Input: part model. Units: mm. Frame: model coordinates. A direction names the side the tool comes from. Coordinates: 2 decimals unless noted, no trailing zeros. Loops run counter-clockwise (first coordinate to the right, second up) from the corner with the lowest first, then second, coordinate; pieces in that order, holes last.
(1) Section B-B, the plane z = 5. Return loops of the section in (x, y), then the cut area to 3 significant figures.
(2) Section C-C, the plane y = -16. Return loops of the section in (x, z), then the cut area to 3 significant figures.
(3) Set-up query: faces 4 (the face through (-31, -13, -23.456)), 5 (the face through (0, -32, 65.444)), 6 (the face through (0, 0.98, 91)). Return all of +Z, -Z, +X, -X, +Y, -Y with unobstructed straight access to the full face (end or side cutting, diameter ignored); none if empty.
(4) Mould query, pull axis Y, two halves, no side actions, for faces 1 (the face through (0, 0, 9)), 2 (the face through (0, -13, -48.856)), 3 (the face through (-13.68, -13, 91)). Classes: released by +Y, released by -Y, zero draft, split by the parting line, or undercut.
(5) Section A-A, the plane x = -2.5. Return loops of the section in (y, z), then the cut area to 3 significant figures.
(6) Line query: L1, parallel to Z at x = 35, y = -22; L2, parallel to Z at x = 25, y = -25; L3, parallel to X at y = -10.5, z = 87.5. Output: solid intervals per line, ascending.
(7) Contact query for flat-ended pins moving along their axis: P1, Ø12, axis at y = -25, z = 89, coming from the -X side; P2, Ø12, axis at x = -7, z = -17, coming from the -Y side; P3, Ø1, axis at y = 8.5, z = 68.5, coming from the +X side. Output: stop coordinate, or through.
```python
from build123d import *

# Parameters (mm, degrees)
F1_DEPTH = 25.4
F2_R     = 7.890546565
F3_DEPTH = 63.501
F5_DEPTH = 50.8
F7_DEPTH = 50.8


with BuildPart() as f1:
    # F0 (on Front) → F1 (new body)
    with BuildSketch(Plane.XZ):
        Polygon((-44.0221392334, -23.4564554393), (-44.0221392334, -48.8564554393), (44.8778607666, -48.8564554393), (44.8778607666, -23.4564554393), (19.4778607666, -23.4564554393), (19.4778607666, 40.0435445607), (44.8778607666, 40.0435445607), (44.8778607666, 65.4435445607), (-44.0221392334, 65.4435445607), (-44.0221392334, 40.0435445607), (-18.6221392334, 40.0435445607), (-18.6221392334, -23.4564554393), align=None)
    extrude(amount=F1_DEPTH)

    # F2 (on face) → F3 (cut, through all)
    with BuildSketch(Plane.YZ.offset(19.4778607666)):
        with Locations((-12.7, 8.2935445607)):
            Circle(F2_R)
    extrude(amount=-F3_DEPTH, mode=Mode.SUBTRACT)

    # F4 (on face) → F5 (join)
    with BuildSketch(Plane.XY.offset(65.4435445607)):
        with BuildLine():
            Line((-27.2401830653, 0), (27.2401830653, 0))
            ThreePointArc((27.2401830653, 0), (0, 17.3552420291), (-27.2401830653, 0))
        make_face()
        with BuildLine():
            ThreePointArc((-27.2401830653, -25.4), (0, -42.7552420291), (27.2401830653, -25.4))
            Line((27.2401830653, -25.4), (-27.2401830653, -25.4))
        make_face()
        with BuildLine():
            ThreePointArc((27.2401830653, -25.4), (29.3430389392, -19.2041247868), (30.0552420291, -12.7))
            ThreePointArc((30.0552420291, -12.7), (29.3430389392, -6.1958752132), (27.2401830653, 0))
            Line((27.2401830653, 0), (-27.2401830653, 0))
            ThreePointArc((-27.2401830653, 0), (-30.0552420291, -12.7), (-27.2401830653, -25.4))
            Line((-27.2401830653, -25.4), (27.2401830653, -25.4))
        make_face()
    extrude(amount=F5_DEPTH)

    # F6 (on face) → F7 (cut)
    with BuildSketch(Plane.XY.offset(116.2435445607)):
        Polygon((13.6795025319, -18.3662354752), (13.6795025319, -7.0337645248), (5.6662354752, 0.9795025319), (-5.6662354752, 0.9795025319), (-13.6795025319, -7.0337645248), (-13.6795025319, -18.3662354752), (-5.6662354752, -26.3795025319), (5.6662354752, -26.3795025319), align=None)
    extrude(amount=-F7_DEPTH, mode=Mode.SUBTRACT)


solid = f1.part
```
Report:
1. outline: (-18.62, -25.4) - (19.48, -25.4) - (19.48, -19.87) - (-18.62, -19.87) - close; (-18.62, -5.53) - (19.48, -5.53) - (19.48, 0) - (-18.62, 0) - close
1. area: 421 mm2
2. outline: (-44.02, -48.86) - (44.88, -48.86) - (44.88, -23.46) - (19.48, -23.46) - (19.48, 1.13) - (-18.62, 1.13) - (-18.62, -23.46) - (-44.02, -23.46) - close; (-44.02, 40.04) - (-18.62, 40.04) - (-18.62, 15.46) - (19.48, 15.46) - (19.48, 40.04) - (44.88, 40.04) - (44.88, 65.44) - (29.87, 65.44) - (29.87, 116.24) - (13.68, 116.24) - (13.68, 65.44) - (-13.68, 65.44) - (-13.68, 116.24) - (-29.87, 116.24) - (-29.87, 65.44) - (-44.02, 65.44) - close
2. area: 8,030 mm2
3. face 4: -X, +Y, -Y
3. face 5: -Z, +X, -X, -Y
3. face 6: +Z, -Z
4. face 1: released by +Y
4. face 2: zero draft
4. face 3: undercut
5. outline: (-42.65, 65.44) - (-26.38, 65.44) - (-26.38, 116.24) - (-42.65, 116.24) - close; (-25.4, -48.86) - (0, -48.86) - (0, 65.44) - (-25.4, 65.44) - close; (0.98, 65.44) - (17.25, 65.44) - (17.25, 116.24) - (0.98, 116.24) - close; hole circle Ø15.78 at (-12.7, 8.29)
5. area: 4,360 mm2
6. L1: z = -48.86 to -23.46, 40.04 to 65.44
6. L2: z = -48.86 to -23.46, 40.04 to 116.24
6. L3: x = -29.97 to -13.68, 13.68 to 29.97
7. P1: stops at x = -29.39
7. P2: stops at y = -25.4
7. P3: stops at x = 21.79
